Can you work these out from the model? Positions are in its coordinate system, mm. A direction names the side the tool comes from. Coordinates: 2 decimals unless noted, no trailing zeros. Return JSON: item names as keys, results as strings. Group by question number.
1) If we section it at A-A, the plane x = 0: State how many separate pieces and enclosed holes the cut face has, then the cut area to 3 significant figures.
2) If I drill on probe 1 along Y at (x, z) = (0, 10); probe 2 along Y at (x, z) = (-121, 15); probe 3 along Z at (x, y) = (-117, 75), over which ranges is the centre line in solid material (lowest first)? Write a range as from..to.
3) For faces 1 (the flat face through (-118, 28, 55.5)), 2 (the cylindrical face through (119.884, 5.276, 57.472)), 3 (the cylindrical face through (20.59, -92.74, 1.16)), 4 (the cylindrical face through (-1.08, 140.12, 8.11)), which set-ups out of +Z, -Z, +X, -X, +Y, -Y let a thin tool reach every point of the face, with its end or its side?
4) For pin 1 (6 mm diameter, centred on y = -44.5, z = 44, fed in from +X); pin 2 (8 mm diameter, centred on y = -31, z = 4, fed in from -X); pin 3 (4 mm diameter, centred on x = 20, z = 36.5, fed in from -Y), each with a flat end and sliding along its axis, tell me the tip position at first contact or that it passes through.
5) Thinking about a two-plate mould opening in Y: for faces 5 (the flat face through (80, -53, -6)), 6 (the cylindrical face through (-33.601, -151.314, 7.895)), 7 (the cylindrical face through (112.39, 4.95, 13.99)), which applies, +Y half, -Y half, draft (parallel to the pull), parting line (faces both ways), or undercut?
from build123d import *

# Parameters (mm, degrees)
SKETCH_1_R          = 155
EXTRUDE_1_DEPTH     = 20
SKETCH_2_R          = 135
EXTRUDE_2_DEPTH     = 40
SKETCH_3_R          = 120
CUT_EXTRUDE_1_DEPTH = 228.266363547
SKETCH_4_R          = 120
SKETCH_4_R_2        = 112.5
EXTRUDE_3_DEPTH     = 15
SKETCH_5_R          = 121.5
SKETCH_5_R_2        = 120
CUT_EXTRUDE_2_DEPTH = 2.5
SKETCH_7_R          = 5
CUT_EXTRUDE_3_DEPTH = 25
SKETCH_9_R          = 120
CUT_EXTRUDE_4_DEPTH = 13
EXTRUDE_START       = 19
SKETCH_10_R         = 120
SKETCH_10_R_2       = 95
EXTRUDE_4_DEPTH     = 19
EXTRUDE_START_2     = -5
SKETCH_12_R         = 95
SKETCH_12_R_2       = 90
EXTRUDE_5_DEPTH     = 5
CUT_EXTRUDE_START   = -4
SKETCH_13_R         = 155
SKETCH_13_R_2       = 135
CUT_EXTRUDE_5_DEPTH = 4
CHAMFER_1_SIZE      = 0.5
SKETCH_14_W         = 1
SKETCH_14_H         = 0.5


with BuildPart() as part:
    # 草图1 → 拉伸1 (new body)
    with BuildSketch(Plane.XY):
        Circle(SKETCH_1_R)
    extrude(amount=EXTRUDE_1_DEPTH)

    # 草图2 → 拉伸2 (add)
    with BuildSketch(Plane.XY.offset(20)):
        Circle(SKETCH_2_R)
    extrude(amount=EXTRUDE_2_DEPTH)

    # 草图3 → 切除-拉伸1 (cut, through all)
    with BuildSketch(Plane(origin=(0, 0, 0), x_dir=(-1, 0, 0), z_dir=(0, 0, -1))):
        Circle(SKETCH_3_R)
    extrude(amount=-CUT_EXTRUDE_1_DEPTH, mode=Mode.SUBTRACT)

    # 草图4 → 拉伸3 (add)
    with BuildSketch(Plane(origin=(0, 0, 0), x_dir=(-1, 0, 0), z_dir=(0, 0, -1))):
        Circle(SKETCH_4_R)
        Circle(SKETCH_4_R_2, mode=Mode.SUBTRACT)
    extrude(amount=-EXTRUDE_3_DEPTH)

    # 草图5 → 切除-拉伸2 (cut)
    with BuildSketch(Plane.XY.offset(53)):
        Circle(SKETCH_5_R)
        with Locations(Location((0, 0, 0), (0, 0, 180))):
            Circle(SKETCH_5_R_2, mode=Mode.SUBTRACT)
    extrude(amount=CUT_EXTRUDE_2_DEPTH, mode=Mode.SUBTRACT)

    # 草图7 → 切除-拉伸3 (cut)
    with BuildSketch(Plane.XY.offset(20)):
        with Locations((72.5, 125.573683549)):
            Circle(SKETCH_7_R)
        with Locations((0, 145)):
            Circle(SKETCH_7_R)
        with Locations((125.573683549, 72.5)):
            Circle(SKETCH_7_R)
        with Locations((145, 0)):
            Circle(SKETCH_7_R)
        with Locations((125.573683549, -72.5)):
            Circle(SKETCH_7_R)
        with Locations((72.5, -125.573683549)):
            Circle(SKETCH_7_R)
        with Locations((0, -145)):
            Circle(SKETCH_7_R)
        with Locations((-72.5, -125.573683549)):
            Circle(SKETCH_7_R)
        with Locations((-125.573683549, -72.5)):
            Circle(SKETCH_7_R)
        with Locations((-145, 0)):
            Circle(SKETCH_7_R)
        with Locations((-125.573683549, 72.5)):
            Circle(SKETCH_7_R)
        with Locations((-72.5, 125.573683549)):
            Circle(SKETCH_7_R)
    extrude(amount=-CUT_EXTRUDE_3_DEPTH, mode=Mode.SUBTRACT)

    # 草图9 → 切除-拉伸4 (cut)
    with BuildSketch(Plane(origin=(0, 0, 0), x_dir=(-1, 0, 0), z_dir=(0, 0, -1))):
        Circle(SKETCH_9_R)
    extrude(amount=-CUT_EXTRUDE_4_DEPTH, mode=Mode.SUBTRACT)

    # 草图10 → 拉伸4 (add)
    with BuildSketch(Plane(origin=(0, 0, 13), x_dir=(-1, 0, 0), z_dir=(0, 0, -1)).offset(EXTRUDE_START)):
        Circle(SKETCH_10_R)
        Circle(SKETCH_10_R_2, mode=Mode.SUBTRACT)
    extrude(amount=-EXTRUDE_4_DEPTH)

    # 草图12 → 拉伸5 (add)
    with BuildSketch(Plane.XY.offset(13).offset(EXTRUDE_START_2)):
        Circle(SKETCH_12_R)
        Circle(SKETCH_12_R_2, mode=Mode.SUBTRACT)
    extrude(amount=EXTRUDE_5_DEPTH)

    # 草图13 → 切除-拉伸5 (cut)
    with BuildSketch(Plane.XY.offset(20).offset(CUT_EXTRUDE_START)):
        Circle(SKETCH_13_R)
        Circle(SKETCH_13_R_2, mode=Mode.SUBTRACT)
    extrude(amount=CUT_EXTRUDE_5_DEPTH, mode=Mode.SUBTRACT)

    # 倒角1
    chamfer_1_edges = [part.edges().sort_by_distance(p)[0] for p in [
        (120, 0, 60),
        (-155, 0, 16),
        (-155, 0, 0),
        (-135, 0, 60),
        (120, 0, -6),
        (95, 0, -6),
    ]]
    chamfer(chamfer_1_edges, length=CHAMFER_1_SIZE)

    # 草图14 → 切除-旋转1 (revolve, cut)
    with BuildSketch(Plane(origin=(0, 0, 0), x_dir=(1, 0, 0), z_dir=(0, 1, 0)), mode=Mode.PRIVATE) as cut_revolve_1_sk:
        with Locations((-135.5, -15.75)):
            Rectangle(SKETCH_14_W, SKETCH_14_H)
    revolve(cut_revolve_1_sk.sketch.rotate(Axis((0, 0, 8), (0, 0, -1)), 180), axis=Axis((0, 0, 8), (0, 0, -1)), mode=Mode.SUBTRACT)


solid = part.part
Result sheet:
{
 "1": {"separate pieces": "4", "enclosed holes": "0", "area": "3,140 mm2"},
 "2": {"probe 1": "y = -155..-150, -140..-90, 90..140, 150..155", "probe 2": "y = -96.87..-74.52, -70.48..70.48, 74.52..96.87", "probe 3": "z = 0..16"},
 "3": {"face 1": "none", "face 2": "+Z", "face 3": "-Z", "face 4": "+Z, -Z"},
 "4": {"pin 1": "stops at x = 128.46", "pin 2": "stops at x = -152.63", "pin 3": "stops at y = -133.79"},
 "5": {"face 5": "draft", "face 6": "parting line", "face 7": "undercut"}
}
